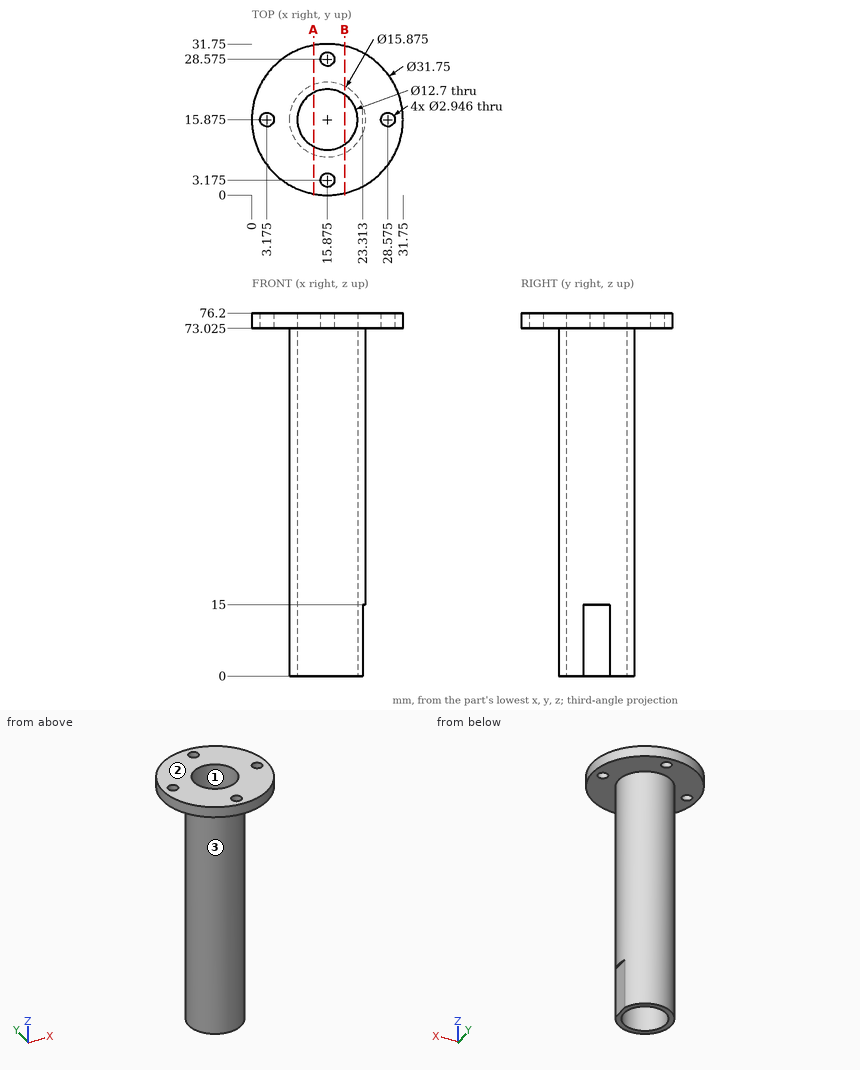
The drawing under review shows one solid part. Ordinate dimensions are in mm from its lowest x, y, z. Coordinates: 2 decimals unless noted, no trailing zeros. Order: outer loops, then holes, each group sorted by start corner. A loop starts at its lowest first (then second) coordinate and runs counter-clockwise, first axis right, second up. Notation, with made-up numbers: (71, 8.5) -> (120, 8.5) arc R20 cw to (120, 27.5) -> close; hole circle Ø4 at (87, 79). An arc over 180 degrees is marked (long way). Answer as CSV lines item,"result".
Q1. We need section A-A (x = 13). State the section outline as (y, z) points (1 decimal).
Model answer:
outline,"(0.3, 73) -> (8.5, 73) -> (8.5, 0) -> (10.2, 0) -> (10.2, 76.2) -> (0.3, 76.2) -> close; (21.5, 0) -> (23.3, 0) -> (23.3, 73) -> (31.5, 73) -> (31.5, 76.2) -> (21.5, 76.2) -> close"
Q2. We need section B-B (x = 19.5). State the section outline as (y, z) points (1 decimal), plus the area to 3 significant figures.
Model answer:
outline,"(0.4, 73) -> (8.8, 73) -> (8.8, 0) -> (10.7, 0) -> (10.7, 76.2) -> (0.4, 76.2) -> close; (21.1, 0) -> (22.9, 0) -> (22.9, 73) -> (31.3, 73) -> (31.3, 76.2) -> (21.1, 76.2) -> close"
area,"335 mm2"
Q3. Wall thickness on line 1 along Z through (x, y) = (29, 18) (1 decimal); line 2 along Y through (x, z) = (18, 50); line 3 along Y through (x, z) = (18.5, 48) (1 decimal): over which ranges is each line inside the solid? List them lowest first. Write a range as [from, to].
Model answer:
line 1,"z = [73, 76.2]"
line 2,"y = [8.23, 9.89], [21.86, 23.52]"
line 3,"y = [8.4, 10.1], [21.7, 23.4]"
Q4. Clearance check with flat-ended pins moving along their axes: pin 1 Ø1.5 at (x, z) = (15.5, 54) entering from +Y; pin 2 Ø2 at (y, z) = (22, 57.5) entering from +X (1 decimal); pin 3 Ø12 at (x, z) = (25.5, 21.5) entering from -Y; pin 4 Ø6 at (y, z) = (4, 45) entering from +X. State where each tip first meets the part, or that it passes through.
Model answer:
pin 1,"stops at y = 23.81"
pin 2,"stops at x = 21.9"
pin 3,"stops at y = 8.81"
pin 4,"passes through"
Q5. Draft analysis for pull direction X (two halves, no side actions). For the marked faces 1, 2 and 3, state which applies: released by +X, released by -X, zero draft, split by the parting line, or undercut.
Model answer:
face 1,"undercut"
face 2,"zero draft"
face 3,"split by the parting line"
